Part model, mm, in its own coordinate system. A direction names the side the tool comes from. Round coordinates to 2 decimals unless told otherwise and drop trailing zeros. Loops run counter-clockwise (first coordinate to the right, second up) from the corner with the lowest first, then second, coordinate; pieces in that order, holes last. Notation, with made-up numbers: (27.5, 61.5) -> (61.5, 61.5) arc R23 ccw to (61.5, 98.5) -> close; hole circle Ø5 at (7.5, 35). An arc over 180 degrees is marked (long way). Use a Markdown table: item, result. Add a question column.
Item 1: Cut at C-C, the plane z = 475.5. List the corners of the cut face in (x, y), plus the area to 3 significant figures.
Item 2: Probe line 1 (Y direction, x = 5, z = 441); line 2 (X direction, y = -16, z = 380); line 3 (Y direction, x = 6.25, z = 481). List the from-to ranges inside material, lowest first. Write a range as [from, to].
Item 3: Cut at A-A, the plane z = 414.5. List the corners of the cut face in (x, y), plus the area to 3 significant figures.
Item 4: Which spindle directions (+Z, -Z, +X, -X, +Y, -Y) get a long thin tool onto all of the face, cutting with end or side? Do faces 1 (the face through (0.5, -0.1, 496.5)), 2 (the face through (6.5, 16, 437)), 3 (the face through (1, -6, 437)). Say none if no direction does.
Item 5: Cut at B-B, the plane y = 0. List the corners of the cut face in (x, z).
Item 6: Flat gauge pins, fed straight in: pin 1 (0.5 mm diameter, centred on x = 0.5, z = 439, fed in from -Y); pin 2 (1 mm diameter, centred on y = -4, z = 476, fed in from -X); pin 3 (1.8 mm diameter, centred on y = -16, z = 452, fed in from -X); pin 4 (1.1 mm diameter, centred on x = 0.5, z = 410, fed in from +Y). Where does each tip first touch, or does it go through?
Item 7: Cut at D-D, the plane y = -7. List the corners of the cut face in (x, z).
Item 8: Two-plate mould, pull along Y, no slides. Class faces 4 (the face through (3, -13.5, 437)), 5 (the face through (0.5, -0.1, 396.5)), 6 (the face through (4, 13.5, 437)): pulls with the +Y half, pulls with the -Y half, needs draft (parallel to the pull), parting line crosses it, or undercut.
```python
from build123d import *

# Parameters (mm, degrees)
BOSS_EXTRUDE1_DEPTH = 500
CUT_EXTRUDE1_DEPTH  = 7.5
LPATTERN1_COUNT     = 40
LPATTERN1_PITCH     = 25
CUT_EXTRUDE2_START  = -127
SKETCH3_W           = 18.151488818
SKETCH3_H           = 38.961529028
CUT_EXTRUDE2_DEPTH  = 874.181233577


with BuildPart() as part:
    # Sketch1 → Boss-Extrude1 (new, symmetric)
    with BuildSketch(Plane.XY):
        with BuildLine():
            Line((7.5, 17.5), (6.5, 17.5))
            Line((6.5, 17.5), (6.5, 14))
            ThreePointArc((6.5, 14), (6.353553391, 13.646446609), (6, 13.5))
            Line((6, 13.5), (1, 13.5))
            ThreePointArc((1, 13.5), (0.292893219, 13.207106781), (0, 12.5))
            Line((0, 12.5), (0, -12.5))
            ThreePointArc((0, -12.5), (0.292893219, -13.207106781), (1, -13.5))
            Line((1, -13.5), (6, -13.5))
            ThreePointArc((6, -13.5), (6.353553391, -13.646446609), (6.5, -14))
            Line((6.5, -14), (6.5, -17.5))
            Line((6.5, -17.5), (7.5, -17.5))
            Line((7.5, -17.5), (7.5, -13.5))
            ThreePointArc((7.5, -13.5), (7.207106781, -12.792893219), (6.5, -12.5))
            Line((6.5, -12.5), (1.5, -12.5))
            ThreePointArc((1.5, -12.5), (1.146446609, -12.353553391), (1, -12))
            Line((1, -12), (1, 12))
            ThreePointArc((1, 12), (1.146446609, 12.353553391), (1.5, 12.5))
            Line((1.5, 12.5), (6.5, 12.5))
            ThreePointArc((6.5, 12.5), (7.207106781, 12.792893219), (7.5, 13.5))
            Line((7.5, 13.5), (7.5, 17.5))
        make_face()
    extrude(amount=BOSS_EXTRUDE1_DEPTH, both=True)

    # Sketch2 → Cut-Extrude1 (cut)
    with BuildSketch(Plane(origin=(0, 0, 0), x_dir=(0, 0, -1), z_dir=(1, 0, 0))):
        with BuildLine():
            Line((-493.35, 3.15), (-481.65, 3.15))
            ThreePointArc((-481.65, 3.15), (-478.5, 0), (-481.65, -3.15))
            Line((-481.65, -3.15), (-493.35, -3.15))
            ThreePointArc((-493.35, -3.15), (-496.5, 0), (-493.35, 3.15))
        make_face()
    cut_extrude1 = extrude(amount=CUT_EXTRUDE1_DEPTH, mode=Mode.SUBTRACT)

    # LPattern1: Cut-Extrude1 ×40
    with Locations(*[(0, 0, -i * LPATTERN1_PITCH) for i in range(1, LPATTERN1_COUNT)]):
        add(cut_extrude1, mode=Mode.SUBTRACT)

    # Sketch3 → Cut-Extrude2 (cut, through all)
    with BuildSketch(Plane.XY.offset(500).offset(CUT_EXTRUDE2_START)):
        with Locations((4.262528883, -0.137511279)):
            Rectangle(SKETCH3_W, SKETCH3_H)
    extrude(amount=-CUT_EXTRUDE2_DEPTH, mode=Mode.SUBTRACT)


solid = part.part
```
A:
| question | item | result |
|---|---|---|
| 1 | outline | (0, -12.5) arc R1 ccw to (1, -13.5) -> (6, -13.5) arc R0.5 cw to (6.5, -14) -> (6.5, -17.5) -> (7.5, -17.5) -> (7.5, -13.5) arc R1 ccw to (6.5, -12.5) -> (1.5, -12.5) arc R0.5 cw to (1, -12) -> (1, 12) arc R0.5 cw to (1.5, 12.5) -> (6.5, 12.5) arc R1 ccw to (7.5, 13.5) -> (7.5, 17.5) -> (6.5, 17.5) -> (6.5, 14) arc R0.5 cw to (6, 13.5) -> (1, 13.5) arc R1 ccw to (0, 12.5) -> close |
| 1 | area | 47.4 mm^2 |
| 2 | line 1 | y = [-13.5, -12.5], [12.5, 13.5] |
| 2 | line 2 | x = [6.5, 7.5] |
| 2 | line 3 | y = [-13.57, -12.5], [12.5, 13.57] |
| 3 | outline | (0, -12.5) arc R1 ccw to (1, -13.5) -> (6, -13.5) arc R0.5 cw to (6.5, -14) -> (6.5, -17.5) -> (7.5, -17.5) -> (7.5, -13.5) arc R1 ccw to (6.5, -12.5) -> (1.5, -12.5) arc R0.5 cw to (1, -12) -> (1, -3.15) -> (0, -3.15) -> close; (0, 3.15) -> (1, 3.15) -> (1, 12) arc R0.5 cw to (1.5, 12.5) -> (6.5, 12.5) arc R1 ccw to (7.5, 13.5) -> (7.5, 17.5) -> (6.5, 17.5) -> (6.5, 14) arc R0.5 cw to (6, 13.5) -> (1, 13.5) arc R1 ccw to (0, 12.5) -> close |
| 3 | area | 41.1 mm^2 |
| 4 | face 1 | +X, -X |
| 4 | face 2 | +Z, -Z, -X, +Y |
| 4 | face 3 | +Z, -Z, +X |
| 5 | outline | (0, 373) -> (1, 373) -> (1, 378.5) -> (0, 378.5) -> close; (0, 396.5) -> (1, 396.5) -> (1, 403.5) -> (0, 403.5) -> close; (0, 421.5) -> (1, 421.5) -> (1, 428.5) -> (0, 428.5) -> close; (0, 446.5) -> (1, 446.5) -> (1, 453.5) -> (0, 453.5) -> close; (0, 471.5) -> (1, 471.5) -> (1, 478.5) -> (0, 478.5) -> close; (0, 496.5) -> (1, 496.5) -> (1, 500) -> (0, 500) -> close |
| 6 | pin 1 | stops at y = -13.47 |
| 6 | pin 2 | stops at x = 0 |
| 6 | pin 3 | stops at x = 6.5 |
| 6 | pin 4 | stops at y = 13.5 |
| 7 | outline | (0, 373) -> (1, 373) -> (1, 500) -> (0, 500) -> close |
| 8 | face 4 | pulls with the -Y half |
| 8 | face 5 | undercut |
| 8 | face 6 | pulls with the +Y half |
